Can you work these out from the drawing? Everything is in mm from the part's minimum corner. A direction names the side the tool comes from. Round coordinates to 2 decimals unless told otherwise and drop trailing zeros. Write each loop counter-clockwise with the first axis right and the second up, starting at its lowest first coordinate (ties: lowest second). Pieces come first, ordered by that corner, then holes. Notation, with made-up numbers: (84, 48) -> (119, 48) arc R26 cw to (119, 65) -> close; hole circle Ø4 at (84, 7). An arc over 180 degrees is marked (long way). Answer as CSV lines item,"result".
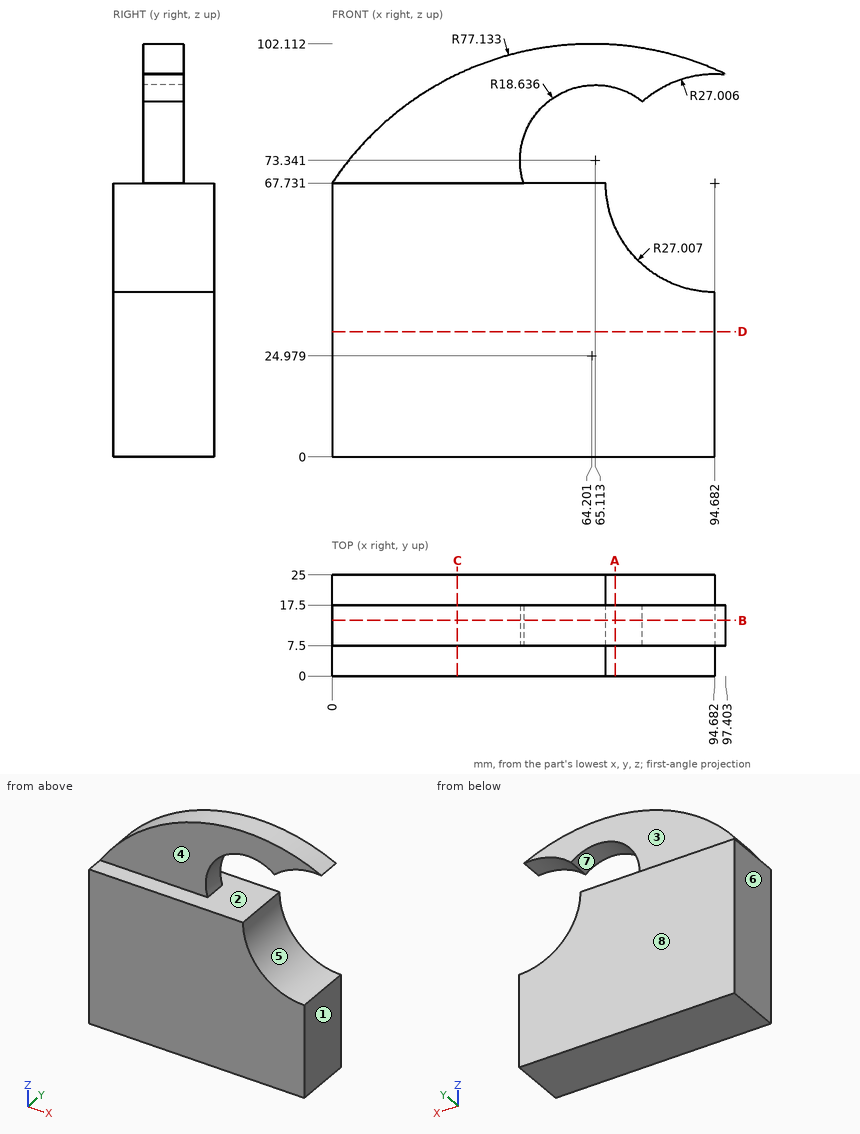
Item 1: If we mould it in two halves opening along X, with no side actions, what happens to the marked faces 5, 6, 7 and 8? For each: pulls with the +X half, pulls with the -X half, needs draft (parallel to the pull), parting line crosses it, or undercut.
Results found:
face 5,"pulls with the +X half"
face 6,"pulls with the -X half"
face 7,"undercut"
face 8,"needs draft"
Item 2: Suppose I cut it at B-B, the plane y = 13.75. List the corners of the cut face in (x, z) for me (1 decimal), then the cut area to 3 significant figures.
Results found:
outline,"(0, 0) -> (94.7, 0) -> (94.7, 40.7) arc R27 cw to (67.7, 67.7) -> (47.3, 67.7) arc R18.6 cw to (76.7, 87.9) arc R27 cw to (97.4, 94.6) arc R77.1 ccw to (0, 67.7) -> close"
area,"7,290 mm²"
Item 3: I need wall thicknesses on L1, parallel to Z at x = 65, y = 11; L2, parallel to Y at x = 40.5, z = 96; L3, parallel to Z at x = 63.5, y = 19. Which ranges of each line are inside material? Lowest first, please.
Results found:
L1,"z = 0 to 67.73, 91.98 to 102.11"
L2,"y = 7.5 to 17.5"
L3,"z = 0 to 67.73"
Item 4: Suppose I cut it at C-C, the plane x = 31. List the corners of the cut face in (y, z) for me, then the cut area to 3 significant figures.
Results found:
outline,"(0, 0) -> (25, 0) -> (25, 67.73) -> (17.5, 67.73) -> (17.5, 94.6) -> (7.5, 94.6) -> (7.5, 67.73) -> (0, 67.73) -> close"
area,"1,960 mm²"
Item 5: Suppose I cut it at D-D, the plane z = 31. List the corners of the cut face in (x, y) for me, then the cut area to 3 significant figures.
Results found:
outline,"(0, 0) -> (94.68, 0) -> (94.68, 25) -> (0, 25) -> close"
area,"2,370 mm²"
Item 6: For the marked faces 1, 2, 3 and 4, which set-ups out of +Z, -Z, +X, -X, +Y, -Y let a thin tool reach every point of the face, with its end or its side?
Results found:
face 1,"-Z, +X, +Y, -Y"
face 2,"+X"
face 3,"+Z, +X, -X, +Y"
face 4,"+Z, +X, -X, -Y"
Item 7: Will these pins go through, and if not, where does the flat tip stop? pin 1 (12.5 mm diameter, centred on x = 25, y = 17.5, fed in from +Z); pin 2 (1.5 mm diameter, centred on y = 21.5, z = 46.5, fed in from +X); pin 3 (2 mm diameter, centred on x = 46.5, y = 20.5, fed in from +Z).
Results found:
pin 1,"stops at z = 94.72"
pin 2,"stops at x = 78.99"
pin 3,"stops at z = 67.73"
Item 8: Suppose I cut it at A-A, the plane x = 70. List the corners of the cut face in (y, z) for me (1 decimal), then the cut area to 4 significant figures.
Results found:
outline,"(0, 0) -> (25, 0) -> (25, 56.8) -> (0, 56.8) -> close; (7.5, 91.3) -> (17.5, 91.3) -> (17.5, 101.9) -> (7.5, 101.9) -> close"
area,"1,525 mm²"
